Geometry check sheet. Reference: the model listing, model coordinates, mm. Give positions to 0.01 mm unless a question says otherwise; leave off trailing zeros. Write each loop counter-clockwise with the first axis right and the second up, starting at its lowest first coordinate (ties: lowest second). Pieces come first, ordered by that corner, then holes. Notation, with made-up numbers: (62.25, -4.75) - (110.25, -4.75) arc R36 cw to (110.25, 30.25) - close; hole circle Ø6 at (39, 41). An arc over 180 degrees is marked (long way). Use a Markdown table: item, result.
```python
from build123d import *

# Parameters (mm, degrees)
ESTRUSIONE_ESTRUSIONE1_DEPTH = 30
SCHIZZO2_R                   = 9.5
TAGLIO_ESTRUSIONE1_DEPTH     = 41.655062299
SMUSSO1_SIZE                 = 1
RACCORDO1_R                  = 1


with BuildPart() as part:
    # Schizzo1 → Estrusione-Estrusione1 (new body)
    with BuildSketch(Plane.XY):
        Polygon((8.03635208, 19.401470183), (-8.03635208, 19.401470183), (-19.401470183, 8.03635208), (-19.401470183, -8.03635208), (-8.03635208, -19.401470183), (8.03635208, -19.401470183), (19.401470183, -8.03635208), (19.401470183, 8.03635208), align=None)
    extrude(amount=ESTRUSIONE_ESTRUSIONE1_DEPTH)

    # Schizzo2 → Taglio-Estrusione1 (cut, through all)
    with BuildSketch(Plane(origin=(0, 0, 0), x_dir=(-1, 0, 0), z_dir=(0, 0, -1))):
        Circle(SCHIZZO2_R)
    extrude(amount=-TAGLIO_ESTRUSIONE1_DEPTH, mode=Mode.SUBTRACT)

    # Smusso1
    smusso1_edges = [part.edges().sort_by_distance(p)[0] for p in [
        (9.5, 0, 30),
        (9.5, 0, 0),
    ]]
    chamfer(smusso1_edges, length=SMUSSO1_SIZE)

    # Raccordo1
    raccordo1_edges = [part.edges().sort_by_distance(p)[0] for p in [
        (19.401470183, 0, 0),
        (13.718911131, -13.718911131, 0),
        (-13.718911131, 13.718911131, 30),
        (0, -19.401470183, 0),
        (-13.718911131, -13.718911131, 0),
        (-19.401470183, 0, 0),
        (-13.718911131, 13.718911131, 0),
        (0, 19.401470183, 0),
        (-19.401470183, 0, 30),
        (-13.718911131, -13.718911131, 30),
        (0, -19.401470183, 30),
        (13.718911131, -13.718911131, 30),
        (19.401470183, 0, 30),
        (13.718911131, 13.718911131, 30),
        (0, 19.401470183, 30),
        (13.718911131, 13.718911131, 0),
    ]]
    fillet(raccordo1_edges, radius=RACCORDO1_R)


solid = part.part
```
1) Depth check by flat-ended pin: P1, Ø6, axis at x = 14, z = 3.5, coming from the +Y side; P2, Ø6, axis at y = 12, z = 25, coming from the -X side; P3, Ø1, axis at x = -12, z = 12.5, coming from the +Y side; P4, Ø17, axis at x = 0, y = 0, coming from the +Z side. Enter the tip coordinate at first touch or a pass-through.
Working result:
| item | result |
|---|---|
| P1 | stops at y = 16.44 |
| P2 | stops at x = -18.44 |
| P3 | stops at y = 15.94 |
| P4 | passes through |
2) Mould release check, pull along Y, two halves, no side actions. Record for faces 1 (the cylindrical face through (0.113, -19.101, 0.285)), 2 (the cylindrical face through (-13.597, 13.438, 29.699)), 3 (the cylindrical face through (-4.38, -8.43, 14.8)), 4 (the cylindrical face through (-19.101, -0.113, 0.285)): pulls with the +Y half, pulls with the -Y half, needs draft (parallel to the pull), parting line crosses it, or undercut.
Working result:
| item | result |
|---|---|
| face 1 | pulls with the -Y half |
| face 2 | pulls with the +Y half |
| face 3 | undercut |
| face 4 | needs draft |
3) Section check C-C on z = 7.5. Record the boundary of the cut face in (x, y).
Working result:
| item | result |
|---|---|
| outline | (-19.4, -8.04) - (-8.04, -19.4) - (8.04, -19.4) - (19.4, -8.04) - (19.4, 8.04) - (8.04, 19.4) - (-8.04, 19.4) - (-19.4, 8.04) - close; hole circle Ø19 at (0, 0) |
4) Material ranges on L1, parallel to Y at x = 0, z = 13; L2, parallel to Y at x = -5, z = 5; L3, parallel to X at y = 4, z = 25, recorded low to high. Write a range as from..to.
Working result:
| item | result |
|---|---|
| L1 | y = -19.4..-9.5, 9.5..19.4 |
| L2 | y = -19.4..-8.08, 8.08..19.4 |
| L3 | x = -19.4..-8.62, 8.62..19.4 |
5) Section check A-A on x = 0. Record the boundary of the cut face in (y, z), then the cut area to 3 significant figures.
Working result:
| item | result |
|---|---|
| outline | (-19.4, 1) arc R1 ccw to (-18.4, 0) - (-10.5, 0) - (-9.5, 1) - (-9.5, 29) - (-10.5, 30) - (-18.4, 30) arc R1 ccw to (-19.4, 29) - close; (9.5, 1) - (10.5, 0) - (18.4, 0) arc R1 ccw to (19.4, 1) - (19.4, 29) arc R1 ccw to (18.4, 30) - (10.5, 30) - (9.5, 29) - close |
| area | 591 mm² |
